from build123d import *

# Parameters (mm, degrees)
BOSS_EXTRUDE2_DEPTH = 4.7625
CUT_EXTRUDE2_DEPTH  = 4.7625
SKETCH3_W           = 5
SKETCH3_H           = 4.7625
CUT_EXTRUDE3_DEPTH  = 4.7625


with BuildPart() as part:
    # Sketch1 → Boss-Extrude2 (new body)
    with BuildSketch(Plane(origin=(0, 0, 0), x_dir=(1, 0, 0), z_dir=(0, 1, 0))):
        Polygon((185.950525, 135.919), (185.950525, 147.9675), (6.09505, 147.968), (5.62377, 147.949), (5.15525, 147.894), (4.6936, 147.803), (4.24021, 147.675), (3.79786, 147.511), (3.37068, 147.314), (2.96003, 147.085), (2.56728, 146.822), (2.19797, 146.529), (1.85208, 146.21), (1.53238, 145.865), (1.24024, 145.495), (0.978408, 145.102), (0.748273, 144.691), (0.551215, 144.264), (0.38723, 143.822), (0.259071, 143.368), (0.168121, 142.907), (0.112999, 142.44), (0.0950846, 141.967), (0.0937066, 6.0923), (0.112999, 5.62102), (0.168121, 5.15387), (0.259071, 4.69085), (0.38723, 4.23746), (0.551215, 3.79511), (0.748273, 3.36793), (0.978408, 2.95727), (1.24024, 2.56453), (1.53238, 2.19659), (1.85208, 1.84933), (2.19797, 1.52962), (2.56728, 1.23748), (2.96003, 0.975653), (3.37068, 0.745518), (3.79786, 0.549836), (4.24021, 0.385851), (4.6936, 0.257693), (5.15525, 0.165365), (5.62377, 0.110243), (6.09505, 0.0909507), (185.950525, 0.0909507), (185.950525, 12.1405), (12.1447, 12.1405), (12.1447, 135.919), align=None)
        Polygon((5.10565, 7.5117), (5.58518, 7.75698), (6.11851, 7.84105), (6.65318, 7.75698), (7.13274, 7.5117), (7.51445, 7.12996), (7.75974, 6.65043), (7.8438, 6.11572), (7.75974, 5.5838), (7.51445, 5.10286), (7.13274, 4.72115), (6.65318, 4.47587), (6.11851, 4.3918), (5.58518, 4.47587), (5.10565, 4.72115), (4.72391, 5.10286), (4.47862, 5.5838), (4.39318, 6.11572), (4.47862, 6.65043), (4.72391, 7.12996), align=None, mode=Mode.SUBTRACT)
        Polygon((124.992, 7.5117), (125.473, 7.75698), (126.007, 7.84105), (126.54, 7.75698), (127.021, 7.5117), (127.403, 7.12996), (127.648, 6.65043), (127.732, 6.11572), (127.648, 5.5838), (127.403, 5.10286), (127.021, 4.72115), (126.54, 4.47587), (126.007, 4.3918), (125.473, 4.47587), (124.992, 4.72115), (124.612, 5.10286), (124.365, 5.5838), (124.281, 6.11572), (124.365, 6.65043), (124.612, 7.12996), align=None, mode=Mode.SUBTRACT)
        Polygon((5.10565, 143.338), (5.58518, 143.583), (6.11851, 143.667), (6.65318, 143.583), (7.13274, 143.338), (7.51445, 142.956), (7.75974, 142.477), (7.8438, 141.942), (7.75974, 141.409), (7.51445, 140.929), (7.13274, 140.547), (6.65318, 140.302), (6.11851, 140.217), (5.58518, 140.302), (5.10565, 140.547), (4.72391, 140.929), (4.47862, 141.409), (4.39318, 141.942), (4.47862, 142.477), (4.72391, 142.956), align=None, mode=Mode.SUBTRACT)
        Polygon((124.992, 143.338), (125.473, 143.583), (126.007, 143.667), (126.54, 143.583), (127.021, 143.338), (127.403, 142.956), (127.648, 142.477), (127.732, 141.942), (127.648, 141.409), (127.403, 140.929), (127.021, 140.547), (126.54, 140.302), (126.007, 140.217), (125.473, 140.302), (124.992, 140.547), (124.612, 140.929), (124.365, 141.409), (124.281, 141.942), (124.365, 142.477), (124.612, 142.956), align=None, mode=Mode.SUBTRACT)
    extrude(amount=BOSS_EXTRUDE2_DEPTH)

    # Sketch2 → Cut-Extrude2 (cut)
    with BuildSketch(Plane(origin=(0, 4.7625, 0), x_dir=(1, 0, 0), z_dir=(0, 1, 0))):
        Polygon((180.950525, 141.94325), (180.950525, 147.9675), (185.950525, 147.9675), (185.950525, 141.94325), (185.950525, 135.919), (180.950525, 135.919), align=None)
    extrude(amount=-CUT_EXTRUDE2_DEPTH, mode=Mode.SUBTRACT)

    # Sketch3 → Cut-Extrude3 (cut)
    with BuildSketch(Plane.XY.offset(-147.9675)):
        with Locations((183.450525, 2.38125)):
            Rectangle(SKETCH3_W, SKETCH3_H)
    extrude(amount=-CUT_EXTRUDE3_DEPTH, mode=Mode.SUBTRACT)


solid = part.part
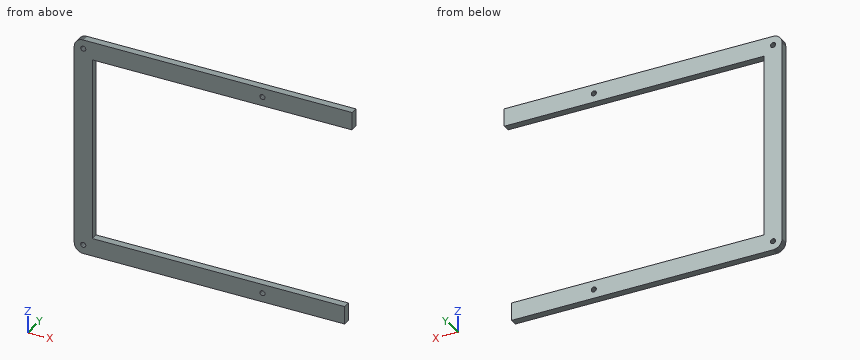
Geometry check sheet. Reference: the model listing, model coordinates, mm. Round coordinates to 2 decimals unless told otherwise and drop trailing zeros. Write each loop counter-clockwise with the first axis right and the second up, starting at its lowest first coordinate (ties: lowest second). Pieces come first, ordered by that corner, then holes.
Item 1: Section check A-A (x = 166.5). Record the boundary of the cut face in (y, z).
Determined:
outline: (0, -147.97) - (4.76, -147.97) - (4.76, -135.92) - (0, -135.92) - close; (0, -12.14) - (4.76, -12.14) - (4.76, -0.09) - (0, -0.09) - close
Item 2: Section check D-D (z = -33). Record the boundary of the cut face in (x, y), plus the area to 3 significant figures.
Determined:
outline: (0.09, 0) - (12.14, 0) - (12.14, 4.76) - (0.09, 4.76) - close
area: 57.4 mm2
Item 3: Section check B-B (y = 2.3). Give the number of separate pieces and of enclosed holes in the cut face, plus the area to 3 significant figures.
Determined:
separate pieces: 1
enclosed holes: 4
area: 5,860 mm2
Item 4: Material ranges on line 1 along Z through (x, y) = (47.5, 0.3); line 2 along X through (y, z) = (3.25, -45.5), recorded low to high.
Determined:
line 1: z = -147.97 to -135.92, -12.14 to -0.09
line 2: x = 0.09 to 12.14
Item 5: Go/stop test with flat-tipped pins: pin 1 Ø1.4 at (y, z) = (2, -55) entering from +X; pin 2 Ø2.5 at (y, z) = (1.5, -143) entering from +X. Record where each tip stops, or that it passes through.
Determined:
pin 1: stops at x = 12.14
pin 2: stops at x = 180.95
